Source: three-view drawing plus pictorial views. Frame: mm from the lowest corner of the part. A direction names the side the tool comes from. Give positions to 0.01 mm unless a question says otherwise; leave off trailing zeros. Order: outer loops, then holes, each group sorted by start corner. A loop starts at its lowest first (then second) coordinate and runs counter-clockwise, first axis right, second up. Notation, with made-up numbers: (-23, 44) - (-12, 44) arc R20 cw to (-12, 69) - close; hole circle Ø7 at (-34, 16). An arc over 180 degrees is marked (long way). Use CSV: the item, a comma, the result in double quotes.
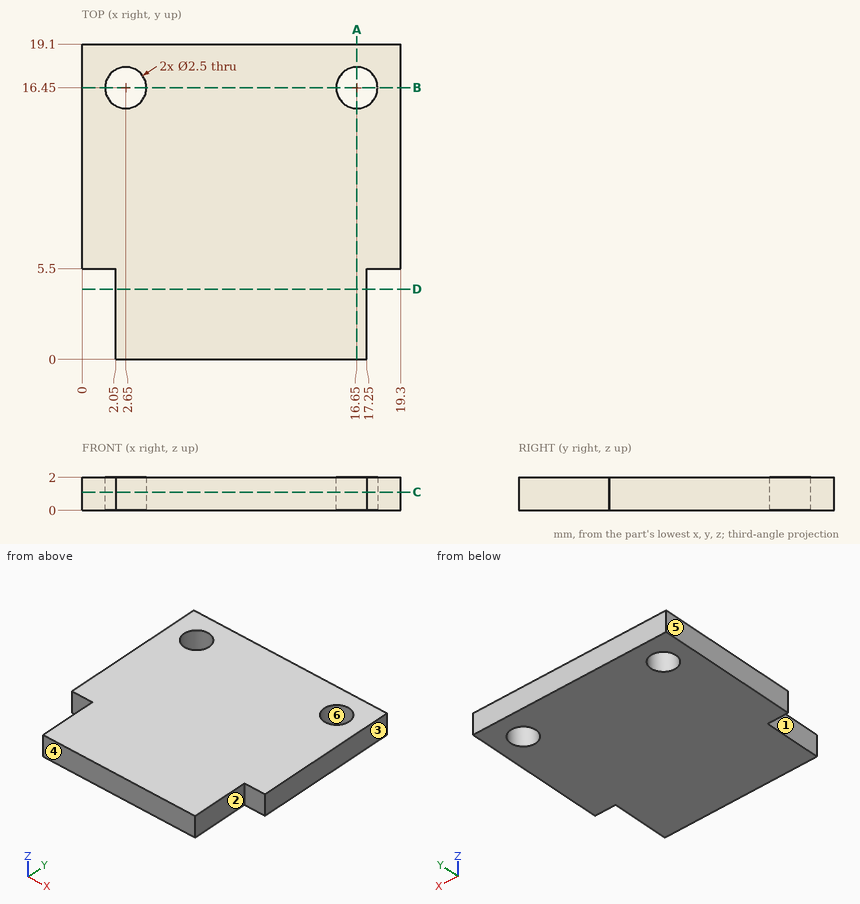
Item 1: Section B-B on y = 16.45. Return the cut outline in (x, z), then the cut area to 3 significant figures.
Filled in:
outline,"(0, 0) - (1.4, 0) - (1.4, 2) - (0, 2) - close; (3.9, 0) - (15.4, 0) - (15.4, 2) - (3.9, 2) - close; (17.9, 0) - (19.3, 0) - (19.3, 2) - (17.9, 2) - close"
area,"28.6 mm2"
Item 2: Section C-C on z = 1.1. Return the cut outline in (x, y), then the cut area to 3 significant figures.
Filled in:
outline,"(0, 5.5) - (2.05, 5.5) - (2.05, 0) - (17.25, 0) - (17.25, 5.5) - (19.3, 5.5) - (19.3, 19.1) - (0, 19.1) - close; hole circle Ø2.5 at (2.65, 16.45); hole circle Ø2.5 at (16.65, 16.45)"
area,"336 mm2"
Item 3: First-contact query: pin 1 (1.5 mm diameter, centred on x = 16.65, y = 16.45, fed in from +Z); pin 2 (1 mm diameter, centred on x = 18.5, z = 1, fed in from -Y); pin 3 (0.6 mm diameter, centred on y = 2.5, z = 0.5, fed in from -X); pin 4 (0.6 mm diameter, centred on y = 2, z = 1, fed in from +X). Flat tips, straight axial feed; report the tip coordinate or a pass-through.
Filled in:
pin 1,"passes through"
pin 2,"stops at y = 5.5"
pin 3,"stops at x = 2.05"
pin 4,"stops at x = 17.25"
Item 4: Section A-A on x = 16.65. Return the cut outline in (y, z).
Filled in:
outline,"(0, 0) - (15.2, 0) - (15.2, 2) - (0, 2) - close; (17.7, 0) - (19.1, 0) - (19.1, 2) - (17.7, 2) - close"
Item 5: Section D-D on y = 4.25. Return the cut outline in (x, z).
Filled in:
outline,"(2.05, 0) - (17.25, 0) - (17.25, 2) - (2.05, 2) - close"
Item 6: Material intervals for line 1 (Y direction, x = 16.65, z = 0.9); line 2 (X direction, y = 1.25, z = 0.1); line 3 (X direction, y = 15.5, z = 0.4), sorted ascending. Write a range as from..to.
Filled in:
line 1,"y = 0..15.2, 17.7..19.1"
line 2,"x = 2.05..17.25"
line 3,"x = 0..1.84, 3.46..15.84, 17.46..19.3"
Item 7: Mould query, pull axis Y, two halves, no side actions, for the marked faces 4, 5 and 6. Classes: released by +Y, released by -Y, zero draft, split by the parting line, or undercut.
Filled in:
face 4,"released by -Y"
face 5,"zero draft"
face 6,"undercut"
Item 8: Set-up query: the marked faces 1, 2 and 3. Return all of +Z, -Z, +X, -X, +Y, -Y with unobstructed straight access to the full face (end or side cutting, diameter ignored); none if empty.
Filled in:
face 1,"+Z, -Z, -X, -Y"
face 2,"+Z, -Z, +X, -Y"
face 3,"+Z, -Z, +X, +Y, -Y"
